```python
from build123d import *

# Parameters (mm, degrees)
BOSS_EXTRUDE1_DEPTH = 9.525
SKETCH3_W           = 14.2875
SKETCH3_H           = 4
CUT_EXTRUDE1_DEPTH  = 22.023216333
SKETCH4_R           = 1.5875
CUT_EXTRUDE2_DEPTH  = 22.023216333


with BuildPart() as part:
    # Sketch1 → Boss-Extrude1 (new body)
    with BuildSketch(Plane(origin=(0, 0, 0), x_dir=(0, 0, -1), z_dir=(1, 0, 0))):
        with BuildLine():
            Line((6.5, 0), (13.5, 0))
            Line((13.5, 0), (13.5, -13))
            Line((13.5, -13), (-13.5, -13))
            Line((-13.5, -13), (-13.5, 0))
            Line((-13.5, 0), (-6.5, 0))
            ThreePointArc((-6.5, 0), (0, -6.5), (6.5, 0))
        make_face()
    extrude(amount=BOSS_EXTRUDE1_DEPTH)

    # Sketch3 → Cut-Extrude1 (cut, through all)
    with BuildSketch(Plane(origin=(9.525, 0, 0), x_dir=(0, 0, -1), z_dir=(1, 0, 0))):
        with Locations((0, -11)):
            Rectangle(SKETCH3_W, SKETCH3_H)
    extrude(amount=-CUT_EXTRUDE1_DEPTH, mode=Mode.SUBTRACT)

    # Sketch4 → Cut-Extrude2 (cut, through all)
    with BuildSketch(Plane.XZ.offset(13)):
        with Locations(Location((4.7625, -10.75, 0), (0, 0, 270))):
            Circle(SKETCH4_R)
        with Locations(Location((4.7625, 10.75, 0), (0, 0, 270))):
            Circle(SKETCH4_R)
    extrude(amount=-CUT_EXTRUDE2_DEPTH, mode=Mode.SUBTRACT)


solid = part.part
```
Read the model definition and answer for the solid it produces. Units are mm, in the model's axes. A direction names the side the tool comes from. Coordinates: 2 decimals unless noted, no trailing zeros. Loops run counter-clockwise (first coordinate to the right, second up) from the corner with the lowest first, then second, coordinate; pieces in that order, holes last. Notation, with made-up numbers: (-34, 86) -> (23, 86) arc R5 ccw to (23, 91) -> close; hole circle Ø6 at (55, -39.5). An arc over 180 degrees is marked (long way). Return JSON: item names as keys, results as strings.
Item 1: Find section B-B (z = 10.75). Determine the outline of the cut face in (x, y) (3 decimals), plus the area to 4 significant figures.
Answers:
{"outline": "(0, -13) -> (3.175, -13) -> (3.175, 0) -> (0, 0) -> close; (6.35, -13) -> (9.525, -13) -> (9.525, 0) -> (6.35, 0) -> close", "area": "82.55 mm2"}
Item 2: Flat-ended cylindrical pins translate along their axes: P1, Ø5, axis at x = 5.5, z = 0.5, coming from the -Y side; P2, Ø3, axis at x = 6.5, z = 1, coming from the +Y side. Find the tip coordinate at first contact, or state that the pin passes through.
Answers:
{"P1": "stops at y = -9", "P2": "stops at y = -6"}
Item 3: For faces 4 (the flat face through (5, -11, 7.144)), 5 (the flat face through (0, -8, 0)), determine the directions among +Z, -Z, +X, -X, +Y, -Y from which every point of the face is accessible in a straight line to the end or side of a thin tool.
Answers:
{"face 4": "+X, -X, -Y", "face 5": "+Z, -Z, -X, +Y, -Y"}
Item 4: Find section A-A (y = -6). Count the separate pieces of the cut face and the enclosed holes in it, plus the area to 3 significant figures.
Answers:
{"separate pieces": "2", "enclosed holes": "2", "area": "194 mm2"}
Item 5: Find section D-D (x = 1.25). Determine the outline of the cut face in (y, z).
Answers:
{"outline": "(-13, -13.5) -> (0, -13.5) -> (0, -6.5) arc R6.5 cw to (0, 6.5) -> (0, 13.5) -> (-13, 13.5) -> (-13, 7.14) -> (-9, 7.14) -> (-9, -7.14) -> (-13, -7.14) -> close"}
Item 6: Find the intervals of material crossed by probe 1 along X at (y, z) = (-8.25, 10.75) (3 decimals); probe 2 along Z at (x, y) = (5.25, -9.75); probe 3 along Z at (x, y) = (5.5, -5), in increasing order.
Answers:
{"probe 1": "x = 0 to 3.175, 6.35 to 9.525", "probe 2": "z = -13.5 to -12.26, -9.24 to -7.14, 7.14 to 9.24, 12.26 to 13.5", "probe 3": "z = -13.5 to -12.16, -9.34 to -4.15, 4.15 to 9.34, 12.16 to 13.5"}
Item 7: Find section C-C (x = 4.25). Determine the outline of the cut face in (y, z), plus the area to 3 significant figures.
Answers:
{"outline": "(-13, -13.5) -> (0, -13.5) -> (0, -12.25) -> (-13, -12.25) -> close; (-13, -9.25) -> (0, -9.25) -> (0, -6.5) arc R6.5 cw to (0, 6.5) -> (0, 9.25) -> (-13, 9.25) -> (-13, 7.14) -> (-9, 7.14) -> (-9, -7.14) -> (-13, -7.14) -> close; (-13, 12.25) -> (0, 12.25) -> (0, 13.5) -> (-13, 13.5) -> close", "area": "149 mm2"}
Item 8: For a pull along X with two mould halves and no side action, classify faces 1 (the cylindrical face through (4.832, -6.591, 12.336)), 2 (the flat face through (5, -7, 13.5)), 3 (the flat face through (9.525, -8, 0)) as +X half, -X half, draft (parallel to the pull), parting line (faces both ways), or undercut.
Answers:
{"face 1": "undercut", "face 2": "draft", "face 3": "+X half"}
